Autodesk Inventor part; units mm, degrees
ref_plane "Work Plane1" through (11.1431, 0, 0) normal (0, 0.7071, -0.7071) x (-1, 0, 0)
ref_plane "YZ Plane" through (0, 0, 0) normal (1, 0, 0) x (0, 1, 0)
ref_plane "XZ Plane" through (0, 0, 0) normal (0, 1, 0) x (-1, 0, 0)
sketch "Sketch1" plane through (0, 0, 0) normal (1, 0, 0) x (0, 1, 0)
  line L0 (0, -3.8891) -> (-3.8891, 0)
  line L1 (-3.8891, 0) -> (0, 3.8891)
  line L2 (0, 3.8891) -> (3.8891, 0)
  line L3 (3.8891, 0) -> (0, -3.8891)
  line L4 (-5.4447, 0) -> (5.4447, 0)
  point P0 (0, 0)
  point P1 (0, 0)
  dimension "d0" = 7.7782
extrude "Body" add sketch "Sketch1" along normal blind 1.78
sketch "Sketch2" plane through (0, 0, 0) normal (-1, 0, 0) x (0, 0, 1)
  point P0 (0, 0)
  point P1 (0, 0)
hole "Thread" at (0, 0, 0) direction (1, 0, 0) diameter 2.459 end through all
chamfer "Chamfer1" distance 0.2706 angle 30 1 edges at (0, 0, -1.2295) measured on face at (0, -1.5681, 1.6031)
chamfer "Chamfer2" distance 0.2706 angle 30 1 edges at (1.78, 0, -1.2295) measured on face at (1.78, -1.5681, 1.6031)
ref_plane "Work Plane1" through (11.1431, 0, 0) normal (0, 0.7071, -0.7071) x (-1, 0, 0)
equation "\"d0\" = 1.41421 * SW"
equation "\"d1\" = KOH"
equation "\"d3\" = -0.5 * GD1 + 0.5 * NND"
equation "\"d35\" = -0.5 * GD1 + 0.5 * NND"
equation "\"d5\" = -0.5 * GD1 + 0.5 * NND"
equation "\"d36\" = -0.5 * GD1 + 0.5 * NND"
equation "\"NND\" = 3"
equation "\"KOH\" = 1.78"
equation "\"SW\" = 5.5"
equation "\"GUL\" = 0.541266 * PTC"
equation "\"THREADDIA\" = 3"
equation "\"TOA\" = 30deg"
equation "\"PTC\" = 0.5"
equation "\"E0\" = 1.155 * SW"
equation "\"GAL\" = 0.541266 * PTC"
properties part number "AS 1474 - M3" material "Steel, Mild"
Input: part model. Units: mm. Frame: model coordinates. Coordinates: 2 decimals unless noted, no trailing zeros. Loops run counter-clockwise (first coordinate to the right, second up) from the corner with the lowest first, then second, coordinate; pieces in that order, holes last. Notation, with made-up numbers: M -32,49 L 16,49 A11 ccw 16,70 Z; hole C -14,-1.5 d8. An arc over 180 degrees is marked long. Use a Markdown table: item, result. Add a question column.
1) Section B-B, the plane z = -3. Return the cut outline in (x, y), plus the area to 3 significant figures.
2) Line query: L1, parallel to Y at x = 1.6, z = -0.25; L2, parallel to Y at x = 0.85, z = -0.75. Output: solid intervals per line, ascending. Write a range as from..to.
3) Section C-C, the plane y = -2. Return the cut outline in (x, z).
4) Section A-A, the plane x = 1.3. Return the cut outline in (y, z).
5) Draft query along Y for faces 1 (the flat face through (0.88, -1.97, 1.92)), 2 (the cylindrical face through (0.9, 0.748, -0.976)), 3 (the flat face through (1.78, -2, 0)). Return one class per face: +Y half, -Y half, draft (parallel to the pull), parting line (faces both ways), or undercut.
Answer below:
| question | item | result |
|---|---|---|
| 1 | outline | M 0,-0.89 L 1.78,-0.89 L 1.78,0.89 L 0,0.89 Z |
| 1 | area | 3.17 mm2 |
| 2 | L1 | -3.64..-1.2, 1.2..3.64 |
| 2 | L2 | -3.14..-0.97, 0.97..3.14 |
| 3 | outline | M 0,-1.89 L 1.78,-1.89 L 1.78,1.89 L 0,1.89 Z |
| 4 | outline | M -3.89,0 L 0,-3.89 L 3.89,0 L 0,3.89 Z; hole C 0,0 d2.46 |
| 5 | face 1 | -Y half |
| 5 | face 2 | undercut |
| 5 | face 3 | draft |
